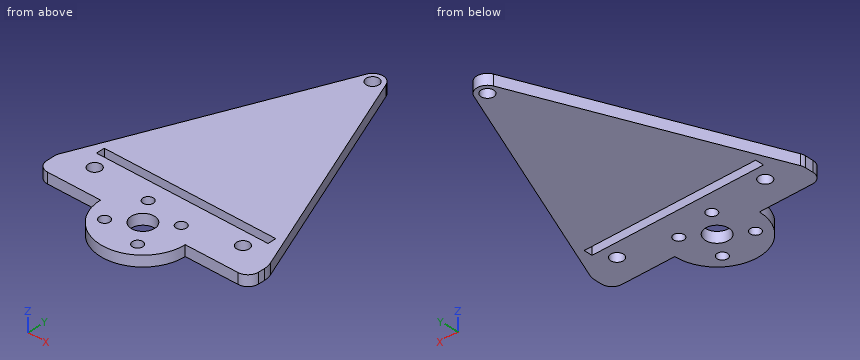
```python
from build123d import *

# Parameters (mm, degrees)
BOSS_EXTRUDE1_DEPTH = 3.175
FILLET4_R           = 3.175
FILLET5_R           = 3.175
FILLET6_R           = 3.175
FILLET7_R           = 6.35
FILLET8_R           = 3.175
SKETCH2_R           = 3.5052
SKETCH2_R_2         = 1.5494
CUT_EXTRUDE1_DEPTH  = 4.175
SKETCH4_W           = 51.435
SKETCH4_H           = 2.54
CUT_EXTRUDE2_DEPTH  = 4.175
SKETCH10_R          = 1.89865
CUT_EXTRUDE3_DEPTH  = 4.175
SKETCH11_R          = 1.89865
CUT_EXTRUDE4_DEPTH  = 4.175


with BuildPart() as part:
    # Sketch1 → Boss-Extrude1 (new body)
    with BuildSketch(Plane.XY):
        with BuildLine():
            Line((-31.75, 0), (-31.75, -6.35))
            Line((-31.75, -6.35), (-12.7, -6.35))
            ThreePointArc((-12.7, -6.35), (0, -19.05), (12.7, -6.35))
            Line((12.7, -6.35), (31.75, -6.35))
            Line((31.75, -6.35), (31.75, 0))
            Line((31.75, 0), (0, 76.2))
            Line((0, 76.2), (-31.75, 0))
        make_face()
    extrude(amount=BOSS_EXTRUDE1_DEPTH)

    # Fillet4
    fillet4_edges = [part.edges().sort_by_distance(p)[0] for p in [
        (-31.75, -6.35, 1.5875),
    ]]
    fillet(fillet4_edges, radius=FILLET4_R)

    # Fillet5
    fillet5_edges = [part.edges().sort_by_distance(p)[0] for p in [
        (-31.75, 0, 1.5875),
    ]]
    fillet(fillet5_edges, radius=FILLET5_R)

    # Fillet6
    fillet6_edges = [part.edges().sort_by_distance(p)[0] for p in [
        (0, 76.2, 1.5875),
    ]]
    fillet(fillet6_edges, radius=FILLET6_R)

    # Fillet7
    fillet7_edges = [part.edges().sort_by_distance(p)[0] for p in [
        (31.75, 0, 1.5875),
    ]]
    fillet(fillet7_edges, radius=FILLET7_R)

    # Fillet8
    fillet8_edges = [part.edges().sort_by_distance(p)[0] for p in [
        (31.75, -6.35, 1.5875),
    ]]
    fillet(fillet8_edges, radius=FILLET8_R)

    # Sketch2 → Cut-Extrude1 (cut, through all)
    with BuildSketch(Plane.XY.offset(3.175)):
        with Locations((0, -6.35)):
            Circle(SKETCH2_R)
        with Locations((-4.880561897, 0.620164745)):
            Circle(SKETCH2_R_2)
        with Locations((4.880561897, -13.320164745)):
            Circle(SKETCH2_R_2)
        with Locations((6.970164745, -1.469438103)):
            Circle(SKETCH2_R_2)
        with Locations((-6.970164745, -11.230561897)):
            Circle(SKETCH2_R_2)
    extrude(amount=-CUT_EXTRUDE1_DEPTH, mode=Mode.SUBTRACT)

    # Sketch4 → Cut-Extrude2 (cut, through all)
    with BuildSketch(Plane.XY.offset(3.175)):
        with Locations((0, 7.634999946)):
            Rectangle(SKETCH4_W, SKETCH4_H)
    extrude(amount=-CUT_EXTRUDE2_DEPTH, mode=Mode.SUBTRACT)

    # Sketch10 → Cut-Extrude3 (cut, through all)
    with BuildSketch(Plane.XY.offset(3.175)):
        with Locations((-22.225, 2.034299946)):
            Circle(SKETCH10_R)
        with Locations((22.225, 2.034299946)):
            Circle(SKETCH10_R)
    extrude(amount=-CUT_EXTRUDE3_DEPTH, mode=Mode.SUBTRACT)

    # Sketch11 → Cut-Extrude4 (cut, through all)
    with BuildSketch(Plane.XY.offset(3.175)):
        with Locations((0, 67.945)):
            Circle(SKETCH11_R)
    extrude(amount=-CUT_EXTRUDE4_DEPTH, mode=Mode.SUBTRACT)


solid = part.part
```
Source: CAD feature listing. Evaluate the final solid. Frame: model axes, mm. Coordinates: 2 decimals unless noted, no trailing zeros. Loops run counter-clockwise (first coordinate to the right, second up) from the corner with the lowest first, then second, coordinate; pieces in that order, holes last. Notation, with made-up numbers: (-30, 19) -> (18, 19) arc R8 cw to (18, 24) -> close; hole circle Ø7 at (79.5, 21.25). An arc over 180 degrees is marked (long way). One line per item, written item: value. Start each with the question number.
Q1. Line query: line 1 along Y through (x, z) = (7.5, 2.4) (3 decimals); line 2 along Y through (x, z) = (6, 1.2) (1 decimal); line 3 along X through (y, z) = (-12.5, 1.4). Output: solid intervals per line, ascending.
Q2. Section query C-C, the plane x = 22. Return the cut outline in (y, z) (3 decimals), and give its area (3 significant figures).
Q3. Section query A-A, the plane x = 14.5. Return the cut outline in (y, z) (3 decimals).
Q4. Contact query for flat-ended pins moving along their axis: P1, Ø1.5, axis at x = -4.5, z = 1, coming from the -Y side; P2, Ø0.8, axis at y = 7.5, z = 1, coming from the -X side; P3, Ø1.6, axis at x = -6.5, z = 2, coming from the +Y side. Output: stop coordinate, or through.
Q5. Section query D-D, the plane y = 48. Return the cut outline in (x, z) (3 decimals), and give its area (3 significant figures).
Q6. Section query B-B, the plane x = 0. Return the cut outline in (y, z) (3 decimals).
Results:
1. line 1: -16.599 to -2.925, -0.013 to 6.365, 8.905 to 58.2
1. line 2: -17.5 to -14.4, -12.2 to -2.7, -0.3 to 6.4, 8.9 to 61.8
1. line 3: -11.11 to -7.86, -6.08 to 3.57, 6.2 to 11.11
2. outline: (-6.35, 0) -> (0.149, 0) -> (0.149, 3.175) -> (-6.35, 3.175) -> close; (3.92, 0) -> (6.365, 0) -> (6.365, 3.175) -> (3.92, 3.175) -> close; (8.905, 0) -> (23.4, 0) -> (23.4, 3.175) -> (8.905, 3.175) -> close
2. area: 74.4 mm^2
3. outline: (-6.35, 0) -> (6.365, 0) -> (6.365, 3.175) -> (-6.35, 3.175) -> close; (8.905, 0) -> (41.4, 0) -> (41.4, 3.175) -> (8.905, 3.175) -> close
4. P1: y = -18.48
4. P2: x = -28.79
4. P3: y = 62.52
5. outline: (-11.75, 0) -> (11.75, 0) -> (11.75, 3.175) -> (-11.75, 3.175) -> close
5. area: 74.6 mm^2
6. outline: (-19.05, 0) -> (-9.855, 0) -> (-9.855, 3.175) -> (-19.05, 3.175) -> close; (-2.845, 0) -> (6.365, 0) -> (6.365, 3.175) -> (-2.845, 3.175) -> close; (8.905, 0) -> (66.046, 0) -> (66.046, 3.175) -> (8.905, 3.175) -> close; (69.844, 0) -> (71.12, 0) -> (71.12, 3.175) -> (69.844, 3.175) -> close
